Read the model definition and answer for the solid it produces. Units are mm, in the model's axes. A direction names the side the tool comes from. Round coordinates to 2 decimals unless told otherwise and drop trailing zeros. Write each loop counter-clockwise with the first axis right and the second up, starting at its lowest first coordinate (ties: lowest second). Pieces come first, ordered by that corner, then holes. Notation, with made-up numbers: (-15, -37) -> (-4, -37) arc R21 ccw to (-4, -25) -> close; hole circle Ø3 at (-29, 85.25). An arc over 180 degrees is marked (long way). Return JSON: item names as keys, results as strings. Group by question number.
(1) Given pin 1 (5.5 mm diameter, centred on x = -21, y = -6, fed in from +Z); pin 2 (6 mm diameter, centred on y = -2, z = 10, fed in from -X); pin 3 (8 mm diameter, centred on y = -5.5, z = 7, fed in from -X), each flat-ended and moving along its own axis, determine where each tip first touches the part or whether it passes through.
(2) The mould has two halves that part along Z. Classify faces 1 (the flat face through (153.363, -7, -2)), 2 (the flat face through (75, -7, 12.49)), 3 (the flat face through (41, -7, 25.858)): released by +Z, released by -Z, zero draft, split by the parting line, or undercut.
(3) For faces 4 (the flat face through (14, -15, -1)), 5 (the flat face through (141.507, -7, 6)), determine the directions among +Z, -Z, +X, -X, +Y, -Y from which every point of the face is accessible in a straight line to the end or side of a thin tool.
(4) A cutting plane is placed at A-A on z = -20. Give the vertices of the cut face in (x, y), then the cut area to 3 significant figures.
(5) A cutting plane is placed at B-B on y = -3.5. State how many separate pieces and enclosed holes the cut face has, then the cut area to 3 significant figures.
(6) Straight lines are drawn through the part: line 1 (Z direction, x = 1.5, y = -8.5); line 2 (Z direction, x = 31, y = -2); line 3 (X direction, y = -4.5, z = 20). For each, find the intervals that lie inside material, in ascending order.
```python
from build123d import *

# Parameters (mm, degrees)
F0_R     = 15.4520785229
F1_DEPTH = 15


with BuildPart() as f1:
    # F0 (on Front) → F1 (new body)
    with BuildSketch(Plane.XZ):
        with BuildLine():
            Line((153.3627957106, 25.8576832712), (-74.0064680576, 25.8576832712))
            Line((-74.0064680576, 25.8576832712), (-74.0064680576, 15.1579529047))
            ThreePointArc((-74.0064680576, 15.1579529047), (-122.2711699364, -0.6687305868), (-74.0064680576, -16.4954140782))
            Line((-74.0064680576, -16.4954140782), (-74.0064680576, -29.4242557138))
            Line((-74.0064680576, -29.4242557138), (153.3627957106, -29.4242557138))
            Line((153.3627957106, -29.4242557138), (153.3627957106, 25.8576832712))
        make_face()
        with Locations((-95.5439214778, -0.6687305868)):
            Circle(F0_R, mode=Mode.SUBTRACT)
        with BuildLine():
            Line((-58.040468074, -16.0495918244), (-58.040468074, 15.7779227399))
            Line((-58.040468074, 15.7779227399), (-49.0474014724, 15.7779227399))
            add(Edge.make_bspline(
                [(-49.0474014724, 15.7779227399), (-42.7153352131, 15.7779227399), (-39.8836686185, 13.8831790407)],
                knots=[0, 0, 0, 1, 1, 1], degree=2))
            add(Edge.make_bspline(
                [(-39.8836686185, 13.8831790407), (-37.052002024, 11.9884353416), (-37.052002024, 7.8994112555)],
                knots=[0, 0, 0, 1, 1, 1], degree=2))
            add(Edge.make_bspline(
                [(-37.052002024, 7.8994112555), (-37.052002024, 5.0642616762), (-38.6297941117, 3.2252457329)],
                knots=[0, 0, 0, 1, 1, 1], degree=2))
            add(Edge.make_bspline(
                [(-38.6297941117, 3.2252457329), (-40.2075861995, 1.3862297896), (-43.2377829242, 0.84288417)],
                knots=[0, 0, 0, 1, 1, 1], degree=2))
            Line((-43.2377829242, 0.84288417), (-43.2377829242, 0.626939116))
            add(Edge.make_bspline(
                [(-43.2377829242, 0.626939116), (-35.9862086932, -0.6130034518), (-35.9862086932, -6.9938314975)],
                knots=[0, 0, 0, 1, 1, 1], degree=2))
            add(Edge.make_bspline(
                [(-35.9862086932, -6.9938314975), (-35.9862086932, -11.2570048206), (-38.8701200589, -13.6532983225)],
                knots=[0, 0, 0, 1, 1, 1], degree=2))
            add(Edge.make_bspline(
                [(-38.8701200589, -13.6532983225), (-41.7540314245, -16.0495918244), (-46.9367127193, -16.0495918244)],
                knots=[0, 0, 0, 1, 1, 1], degree=2))
            Line((-46.9367127193, -16.0495918244), (-58.040468074, -16.0495918244))
        make_face(mode=Mode.SUBTRACT)
        with BuildLine():
            Line((-18.80812795, -2.8142498082), (-25.4536628361, -2.8142498082))
            Line((-25.4536628361, -2.8142498082), (-25.4536628361, -16.0495918244))
            Line((-25.4536628361, -16.0495918244), (-29.1525926312, -16.0495918244))
            Line((-29.1525926312, -16.0495918244), (-29.1525926312, 15.7779227399))
            Line((-29.1525926312, 15.7779227399), (-20.4242328699, 15.7779227399))
            add(Edge.make_bspline(
                [(-20.4242328699, 15.7779227399), (-14.5658525354, 15.7779227399), (-11.7690157883, 13.5348805666)],
                knots=[0, 0, 0, 1, 1, 1], degree=2))
            add(Edge.make_bspline(
                [(-11.7690157883, 13.5348805666), (-8.9721790411, 11.2918383933), (-8.9721790411, 6.7848561383)],
                knots=[0, 0, 0, 1, 1, 1], degree=2))
            add(Edge.make_bspline(
                [(-8.9721790411, 6.7848561383), (-8.9721790411, 0.4736877874), (-15.3739049953, -1.7484564774)],
                knots=[0, 0, 0, 1, 1, 1], degree=2))
            Line((-15.3739049953, -1.7484564774), (-6.7291368679, -16.0495918244))
            Line((-6.7291368679, -16.0495918244), (-11.1037657027, -16.0495918244))
            Line((-11.1037657027, -16.0495918244), (-18.80812795, -2.8142498082))
        make_face(mode=Mode.SUBTRACT)
        with BuildLine():
            Line((18.7384475592, 15.7779227399), (22.4373773542, 15.7779227399))
            Line((22.4373773542, 15.7779227399), (22.4373773542, -4.8134830496))
            add(Edge.make_bspline(
                [(22.4373773542, -4.8134830496), (22.4373773542, -10.2608711847), (19.1494397586, -13.3746595432)],
                knots=[0, 0, 0, 1, 1, 1], degree=2))
            add(Edge.make_bspline(
                [(19.1494397586, -13.3746595432), (15.861502163, -16.4884479018), (10.1145773402, -16.4884479018)],
                knots=[0, 0, 0, 1, 1, 1], degree=2))
            add(Edge.make_bspline(
                [(10.1145773402, -16.4884479018), (4.3676525173, -16.4884479018), (1.2225172961, -13.35027865)],
                knots=[0, 0, 0, 1, 1, 1], degree=2))
            add(Edge.make_bspline(
                [(1.2225172961, -13.35027865), (-1.9226179251, -10.2121093983), (-1.9226179251, -4.7298914158)],
                knots=[0, 0, 0, 1, 1, 1], degree=2))
            Line((-1.9226179251, -4.7298914158), (-1.9226179251, 15.7779227399))
            Line((-1.9226179251, 15.7779227399), (1.7832778394, 15.7779227399))
            Line((1.7832778394, 15.7779227399), (1.7832778394, -4.9876322866))
            add(Edge.make_bspline(
                [(1.7832778394, -4.9876322866), (1.7832778394, -8.9721668305), (3.9601433026, -11.1072364768)],
                knots=[0, 0, 0, 1, 1, 1], degree=2))
            add(Edge.make_bspline(
                [(3.9601433026, -11.1072364768), (6.1370087658, -13.2423061231), (10.358386272, -13.2423061231)],
                knots=[0, 0, 0, 1, 1, 1], degree=2))
            add(Edge.make_bspline(
                [(10.358386272, -13.2423061231), (14.3847166328, -13.2423061231), (16.561582096, -11.0967875225)],
                knots=[0, 0, 0, 1, 1, 1], degree=2))
            add(Edge.make_bspline(
                [(16.561582096, -11.0967875225), (18.7384475592, -8.951268922), (18.7384475592, -4.9458364697)],
                knots=[0, 0, 0, 1, 1, 1], degree=2))
            Line((18.7384475592, -4.9458364697), (18.7384475592, 15.7779227399))
        make_face(mode=Mode.SUBTRACT)
        with BuildLine():
            Line((55.7207795403, 15.7779227399), (55.7207795403, -16.0495918244))
            Line((55.7207795403, -16.0495918244), (51.4994020341, -16.0495918244))
            Line((51.4994020341, -16.0495918244), (34.105376237, 10.6579351705))
            Line((34.105376237, 10.6579351705), (33.9312269999, 10.6579351705))
            add(Edge.make_bspline(
                [(33.9312269999, 10.6579351705), (34.279525474, 5.95590577), (34.279525474, 2.0410309209)],
                knots=[0, 0, 0, 1, 1, 1], degree=2))
            Line((34.279525474, 2.0410309209), (34.279525474, -16.0495918244))
            Line((34.279525474, -16.0495918244), (30.8592344582, -16.0495918244))
            Line((30.8592344582, -16.0495918244), (30.8592344582, 15.7779227399))
            Line((30.8592344582, 15.7779227399), (35.0388161476, 15.7779227399))
            Line((35.0388161476, 15.7779227399), (52.3910461278, -10.8251147127))
            Line((52.3910461278, -10.8251147127), (52.5651953649, -10.8251147127))
            add(Edge.make_bspline(
                [(52.5651953649, -10.8251147127), (52.523399548, -10.2399732762), (52.3701482194, -7.0495592534)],
                knots=[0, 0, 0, 1, 1, 1], degree=2))
            add(Edge.make_bspline(
                [(52.3701482194, -7.0495592534), (52.2168968908, -3.8591452305), (52.2586927077, -2.4868492425)],
                knots=[0, 0, 0, 1, 1, 1], degree=2))
            Line((52.2586927077, -2.4868492425), (52.2586927077, 15.7779227399))
            Line((52.2586927077, 15.7779227399), (55.7207795403, 15.7779227399))
        make_face(mode=Mode.SUBTRACT)
        Polygon((82.2123614812, -12.7407563204), (82.2123614812, -16.0495918244), (64.47003721, -16.0495918244), (64.47003721, 15.7779227399), (82.2123614812, 15.7779227399), (82.2123614812, 12.4899851443), (68.1689670051, 12.4899851443), (68.1689670051, 2.2360780664), (81.3625132044, 2.2360780664), (81.3625132044, -1.0309616207), (68.1689670051, -1.0309616207), (68.1689670051, -12.7407563204), align=None, mode=Mode.SUBTRACT)
        Polygon((113.0994701655, -16.0495918244), (109.2681869502, -16.0495918244), (105.3045503148, -5.9280381667), (92.5498601929, -5.9280381667), (88.6349853439, -16.0495918244), (84.8872937624, -16.0495918244), (97.4678346473, 15.9102761601), (100.5816230059, 15.9102761601), align=None, mode=Mode.SUBTRACT)
        with BuildLine():
            Line((137.8077639189, 15.7779227399), (141.506693714, 15.7779227399))
            Line((141.506693714, 15.7779227399), (141.506693714, -4.8134830496))
            add(Edge.make_bspline(
                [(141.506693714, -4.8134830496), (141.506693714, -10.2608711847), (138.2187561184, -13.3746595432)],
                knots=[0, 0, 0, 1, 1, 1], degree=2))
            add(Edge.make_bspline(
                [(138.2187561184, -13.3746595432), (134.9308185228, -16.4884479018), (129.1838936999, -16.4884479018)],
                knots=[0, 0, 0, 1, 1, 1], degree=2))
            add(Edge.make_bspline(
                [(129.1838936999, -16.4884479018), (123.4369688771, -16.4884479018), (120.2918336559, -13.35027865)],
                knots=[0, 0, 0, 1, 1, 1], degree=2))
            add(Edge.make_bspline(
                [(120.2918336559, -13.35027865), (117.1466984346, -10.2121093983), (117.1466984346, -4.7298914158)],
                knots=[0, 0, 0, 1, 1, 1], degree=2))
            Line((117.1466984346, -4.7298914158), (117.1466984346, 15.7779227399))
            Line((117.1466984346, 15.7779227399), (120.8525941992, 15.7779227399))
            Line((120.8525941992, 15.7779227399), (120.8525941992, -4.9876322866))
            add(Edge.make_bspline(
                [(120.8525941992, -4.9876322866), (120.8525941992, -8.9721668305), (123.0294596624, -11.1072364768)],
                knots=[0, 0, 0, 1, 1, 1], degree=2))
            add(Edge.make_bspline(
                [(123.0294596624, -11.1072364768), (125.2063251256, -13.2423061231), (129.4277026318, -13.2423061231)],
                knots=[0, 0, 0, 1, 1, 1], degree=2))
            add(Edge.make_bspline(
                [(129.4277026318, -13.2423061231), (133.4540329925, -13.2423061231), (135.6308984557, -11.0967875225)],
                knots=[0, 0, 0, 1, 1, 1], degree=2))
            add(Edge.make_bspline(
                [(135.6308984557, -11.0967875225), (137.8077639189, -8.951268922), (137.8077639189, -4.9458364697)],
                knots=[0, 0, 0, 1, 1, 1], degree=2))
            Line((137.8077639189, -4.9458364697), (137.8077639189, 15.7779227399))
        make_face(mode=Mode.SUBTRACT)
    extrude(amount=F1_DEPTH)


solid = f1.part
```
Checks:
{
 "1": {"pin 1": "stops at z = 25.86", "pin 2": "stops at x = -121.15", "pin 3": "stops at x = -122.02"},
 "2": {"face 1": "zero draft", "face 2": "undercut", "face 3": "released by +Z"},
 "3": {"face 4": "+Z, -Z, +X, -X, -Y", "face 5": "+Y, -Y"},
 "4": {"outline": "(-114, -15) -> (-77.09, -15) -> (-77.09, 0) -> (-114, 0) -> close; (-74.01, -15) -> (153.36, -15) -> (153.36, 0) -> (-74.01, 0) -> close", "area": "3,960 mm^2"},
 "5": {"separate pieces": "1", "enclosed holes": "8", "area": "11,400 mm^2"},
 "6": {"line 1": "z = -29.42 to -13.62, 15.78 to 25.86", "line 2": "z = -29.42 to -16.05, 15.78 to 25.86", "line 3": "x = -112.49 to -78.6, -74.01 to 153.36"}
}
